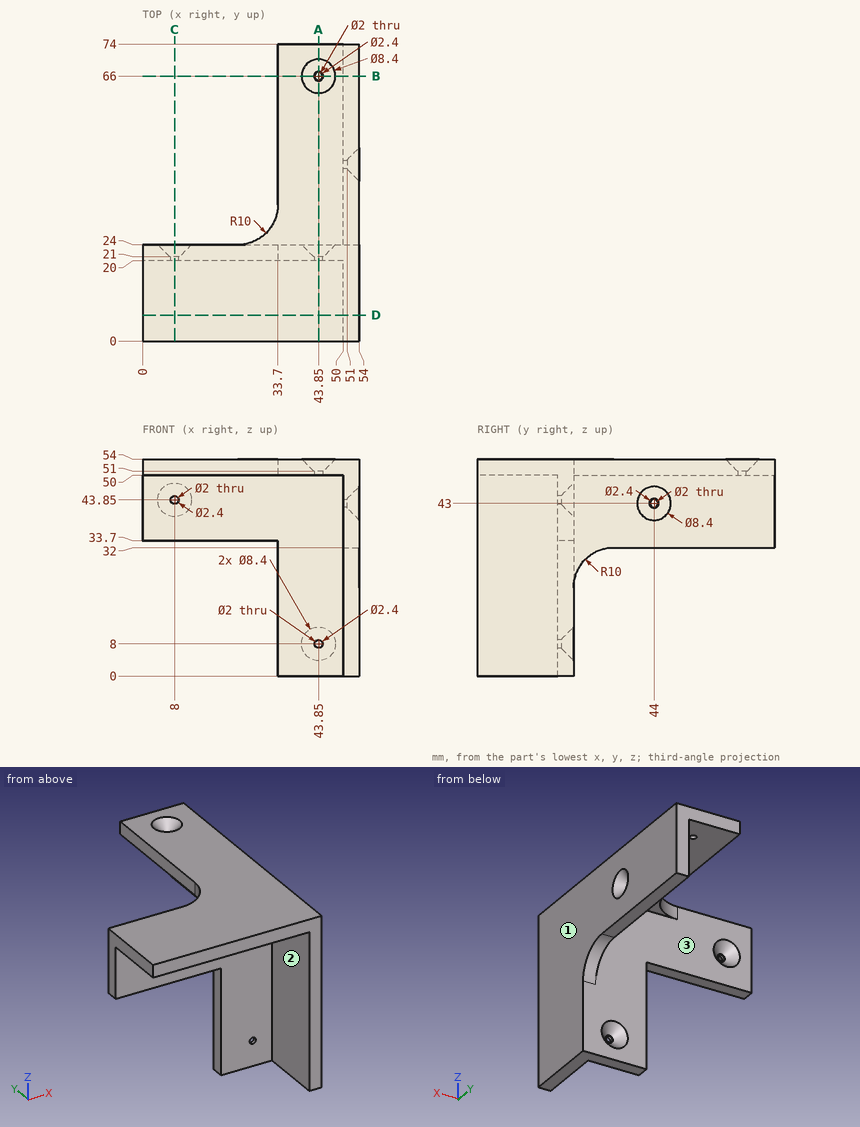
Source: three-view drawing plus pictorial views. Frame: mm from the lowest corner of the part. A direction names the side the tool comes from. Round coordinates to 2 decimals unless told otherwise and drop trailing zeros. Loops run counter-clockwise (first coordinate to the right, second up) from the corner with the lowest first, then second, coordinate; pieces in that order, holes last. Notation, with made-up numbers: M 71.5,10.5 L 118.5,10.5 A25 ccw 118.5,46.5 Z; hole C -8.5,15 d3. An arc over 180 degrees is marked long. Put each result on its own line as item: value. Start each with the question number.
(1) Section query C-C (x = 8). Return loops of the section in (y, z), then the cut area to 3 significant figures.
(2) Section query B-B (y = 66). Return loops of the section in (x, z), then the cut area to 3 significant figures.
(3) Section query D-D (y = 6.5). Return loops of the section in (x, z), then the cut area to 3 significant figures.
(4) Set-up query: the marked faces 1, 2 and 3. Return all of +Z, -Z, +X, -X, +Y, -Y with unobstructed straight access to the full face (end or side cutting, diameter ignored); none if empty.
(5) Contact query for flat-ended pins moving along their axis: pin 1 Ø3 at (x, z) = (10.5, 37) entering from +Y; pin 2 Ø2 at (x, y) = (21.5, 21.5) entering from -Z; pin 3 Ø1.2 at (y, z) = (43.5, 43) entering from +X. Output: stop coordinate, or through.
(6) Section query A-A (x = 43.85). Return loops of the section in (y, z).
(7) Material intervals for line 1 along X through (y, z) = (66, 50.3); line 2 along Y through (x, z) = (43.85, 50.7); line 3 along Z through (x, y) = (46.5, 46.5), sorted ascending. Write a range as [from, to].
Findings below:
1. outline: M 0,50 L 20,50 L 20,44.85 L 21,44.85 L 21,45.05 L 24,48.05 L 24,54 L 0,54 Z; M 20,33.7 L 24,33.7 L 24,39.65 L 21,42.65 L 21,42.85 L 20,42.85 Z
1. area: 143 mm2
2. outline: M 33.7,50 L 42.85,50 L 42.85,51 L 42.65,51 L 39.65,54 L 33.7,54 Z; M 44.85,50 L 50,50 L 50,32 L 54,32 L 54,54 L 48.05,54 L 45.05,51 L 44.85,51 Z
2. area: 135 mm2
3. outline: M 0,50 L 50,50 L 50,0 L 54,0 L 54,54 L 0,54 Z
3. area: 416 mm2
4. face 1: +Z, -Z, +X, +Y, -Y
4. face 2: -Z, -X, -Y
4. face 3: -Z, -X, +Y
5. pin 1: stops at y = 24
5. pin 2: stops at z = 33.7
5. pin 3: stops at x = 51
6. outline: M 0,50 L 20,50 L 20,9 L 21,9 L 21,9.2 L 24,12.2 L 24,50 L 65,50 L 65,51 L 64.8,51 L 61.8,54 L 0,54 Z; M 20,0 L 24,0 L 24,3.8 L 21,6.8 L 21,7 L 20,7 Z; M 67,50 L 74,50 L 74,54 L 70.2,54 L 67.2,51 L 67,51 Z
7. line 1: x = [33.7, 42.85], [44.85, 54]
7. line 2: y = [0, 65], [67, 74]
7. line 3: z = [50, 54]
